from build123d import *

# Parameters (mm, degrees)
PAD_DEPTH     = 20
SKETCH001_R   = 1.65
HOLE_DEPTH    = 10
HOLE_TIPS_R   = 1.65
SKETCH002_R   = 1.65
HOLE001_DEPTH = 20.001


with BuildPart() as part:
    # Sketch → Pad (new body)
    with BuildSketch(Plane.XY):
        Polygon((-65, 0), (-85, 0), (-85, 4.4), (-69.4, 20), (-65, 20), align=None)
    extrude(amount=PAD_DEPTH)

    # Sketch001 (on Face1 of Pad) → Hole (cut)
    with BuildSketch(Plane.XZ):
        with Locations((-75, 10)):
            Circle(SKETCH001_R)
    extrude(amount=-HOLE_DEPTH, mode=Mode.SUBTRACT)

    # Hole tips → Hole tip 1 section 0
    with BuildSketch(Plane.XZ.offset(-10), mode=Mode.PRIVATE) as hole_tip_1_s0:
        with Locations((-75, 10)):
            Circle(HOLE_TIPS_R)
    loft([hole_tip_1_s0.sketch, Vertex(-75, 10.99142, 10)], mode=Mode.SUBTRACT)

    # Sketch002 (on Face4 of Hole) → Hole001 (cut, through all)
    with BuildSketch(Plane.XY.offset(20)):
        with Locations((-70, 10)):
            Circle(SKETCH002_R)
    extrude(amount=-HOLE001_DEPTH, mode=Mode.SUBTRACT)


solid = part.part
Design review of the part built by this model. Coordinates are the model's own, in mm. A direction names the side the tool comes from. Give positions to 0.01 mm unless a question says otherwise; leave off trailing zeros. Write each loop counter-clockwise with the first axis right and the second up, starting at its lowest first coordinate (ties: lowest second). Pieces come first, ordered by that corner, then holes. Notation, with made-up numbers: M 46,31 L 53,31 A22 ccw 53,46 Z; hole C -38.75,8 d1. An arc over 180 degrees is marked long. Answer as a JSON object with one key per item and string values. Group by question number.
1) We need section C-C (z = 3.25). Give the boundary of the cut face in (x, y), and give its area (3 significant figures).
2) Tool access review of faces 1 (the face through (-76.65, 4.93, 10.07)), 2 (the face through (-67, 20, 10)): name each direction out of +Z, -Z, +X, -X, +Y, -Y from which nothing blocks a thin tool from reaching the whole face with its end or side.
3) We need section D-D (y = 12.5). Give the boundary of the cut face in (x, z), and give its area (3 significant figures).
4) For line 1 along Z through (x, y) = (-75, 5.75); line 2 along Y through (x, z) = (-70, 10.5); line 3 along Y through (x, z) = (-69.25, 3.5), list the stretches that pass through material, from the lowest coordinate up.
5) We need section B-B (x = -70). Give the boundary of the cut face in (y, z).
6) Clearance check with flat-ended pins moving along their axes: pin 1 Ø2 at (x, z) = (-75, 10) entering from +Y; pin 2 Ø12 at (y, z) = (13.5, 5) entering from -X; pin 3 Ø1.5 at (x, z) = (-70.5, 10) entering from +Y. State where each tip first meets the part, or that it passes through.
7) Mouldability with a two-part tool opening along X and no side actions: class faces 3 (the face through (-75.263, 10.833, 10.012)), 4 (the face through (-73, 8, 0)), 5 (the face through (-77.3, 12.1, 9.9)) as released by +X, released by -X, zero draft, split by the parting line, or undercut.
8) We need section A-A (y = 9). Give the boundary of the cut face in (x, z), and give its area (3 significant figures).
Answer key:
{
 "1": {"outline": "M -85,0 L -65,0 L -65,20 L -69.4,20 L -85,4.4 Z; hole C -70,10 d3.3", "area": "270 mm²"},
 "2": {"face 1": "-Y", "face 2": "+Z, -Z, +X, -X, +Y"},
 "3": {"outline": "M -76.9,0 L -65,0 L -65,20 L -76.9,20 Z", "area": "238 mm²"},
 "4": {"line 1": "z = 0 to 8.35, 11.65 to 20", "line 2": "y = 0 to 8.35, 11.65 to 19.4", "line 3": "y = 0 to 8.53, 11.47 to 20"},
 "5": {"outline": "M 0,0 L 8.35,0 L 8.35,20 L 0,20 Z; M 11.65,0 L 19.4,0 L 19.4,20 L 11.65,20 Z"},
 "6": {"pin 1": "stops at y = 15.4", "pin 2": "stops at x = -81.9", "pin 3": "stops at y = 19.65"},
 "7": {"face 3": "undercut", "face 4": "zero draft", "face 5": "released by -X"},
 "8": {"outline": "M -80.4,0 L -71.31,0 L -71.31,20 L -80.4,20 Z; M -68.69,0 L -65,0 L -65,20 L -68.69,20 Z; hole C -75,10 d3.3", "area": "247 mm²"}
}
